Verification items for the finished model (mm, model axes). Face numbers are marked on the shaded views. A direction names the side the tool comes from. Give positions to 0.01 mm unless a question says otherwise; leave off trailing zeros. Loops run counter-clockwise (first coordinate to the right, second up) from the corner with the lowest first, then second, coordinate; pieces in that order, holes last. Notation, with made-up numbers: (16, 37.25) -> (70, 37.25) arc R33 cw to (70, 67.25) -> close; hole circle Ø7 at (44, 56.25). An arc over 180 degrees is marked (long way). Answer in a Markdown table with one row per item. Add a question column.
Q1. Material ranges on probe 1 along X at (y, z) = (38.5, 70.5); probe 2 along Y at (x, z) = (12, 71.6); probe 3 along Z at (x, y) = (-9, 7.5), recorded low to high.
Q2. Section check A-A on y = 8.5. Enter the section's corners in (x, z), and give its area (3 significant figures).
Q3. Section check B-B on x = 12. Enter the section's corners in (y, z), and give its area (3 significant figures).
Q4. Section check C-C on x = 3.5. Enter the section's corners in (y, z).
Q5. Set-up check for the marked faces 5, 6, 7, 8 and 9: record each of +Z, -Z, +X, -X, +Y, -Y from which the full face is reachable in a straight line by a thin tool's end or side.
Q6. Release check for a two-part mould opening along Z. For the marked faces 1, 2, 3 and 4 record: pulls with the +Z half, pulls with the -Z half, needs draft (parallel to the pull), parting line crosses it, or undercut.
Q7. Gauge pin test, flat ends, axial feed: P1, Ø3, axis at x = -13.75, y = 31.4, coming from the -Z side; P2, Ø15, axis at x = -4, y = 12.5, coming from the +Z side; P3, Ø1.5, axis at y = 12.5, z = 67, coming from the +X side; P4, Ø1.4, axis at x = -5.5, z = 71.5, coming from the +Y side. Record the tip position at first contact, or that the pin passes through.
Q8. Section check D-D on z = 61.5. Enter the section's corners in (x, y), and give its area (3 significant figures).
Autodesk Inventor part; units mm, degrees
ref_plane "РабПлоскость2" through (-11.5, 28.8975, 52.6492) normal (0, 0, -1) x (0, 1, 0)
ref_plane "РабПлоскость3" through (-11.5, 28.8975, 52.6492) normal (0, 0, -1) x (0, 1, 0)
ref_plane "РабПлоскость4" through (-15, 28.8975, 52.6492) normal (0, -1, 0) x (1, 0, 0)
ref_plane "РабПлоскость1" through (0, 34.8975, 74.4992) normal (0, 0, -1) x (1, 0, 0)
sketch "Эскиз1" plane through (0, 34.8975, 74.4992) normal (0, 0, -1) x (1, 0, 0)
  line L0 (11.5, 6) -> (11.5, -6)
  line L1 (15, -6) -> (11.5, -6)
  arc A0 (15, -6) -> (16, -5) centre (15, -5) ccw
  line L2 (16, -1.25) -> (16, -5)
  line L3 (14, -1.25) -> (16, -1.25)
  arc A1 (12.8, -0.05) -> (14, -1.25) centre (14, -0.05) ccw
  line L4 (12.8, 0.05) -> (12.8, -0.05)
  arc A2 (14, 1.25) -> (12.8, 0.05) centre (14, 0.05) ccw
  line L5 (16, 1.25) -> (14, 1.25)
  line L6 (16, 5) -> (16, 1.25)
  arc A3 (16, 5) -> (15, 6) centre (15, 5) ccw
  line L7 (11.5, 6) -> (15, 6)
  circle A4 centre (13.75, 3.5) radius 1.25
  circle A5 centre (13.75, -3.5) radius 1.25
  line L8 (-11.5, -6) -> (-11.5, 6)
  line L9 (-15, 6) -> (-11.5, 6)
  arc A6 (-15, 6) -> (-16, 5) centre (-15, 5) ccw
  line L10 (-16, 1.3872) -> (-16, 5)
  line L11 (-14, 1.3872) -> (-16, 1.3872)
  arc A7 (-12.802, 0.1186) -> (-14, 1.3872) centre (-14, 0.1872) ccw
  line L12 (-12.802, 0.0186) -> (-12.802, 0.1186)
  arc A8 (-14, -1.25) -> (-12.802, 0.0186) centre (-14, -0.05) ccw
  line L13 (-16, -1.25) -> (-14, -1.25)
  line L14 (-16, -5) -> (-16, -1.25)
  arc A9 (-16, -5) -> (-15, -6) centre (-15, -5) ccw
  line L15 (-11.5, -6) -> (-15, -6)
  circle A10 centre (-13.75, 3.5) radius 1.25
  circle A11 centre (-13.75, -3.5) radius 1.25
  line L16 (16, 5) -> (16, 6)
  line L17 (16, 6) -> (15, 6)
  line L18 (-16, 5) -> (-16, 6)
  line L19 (-16, 6) -> (-15, 6)
  point P0 (0, 34.8975)
extrude "Выдавливание1" add sketch "Эскиз1" along normal blind 6
sketch "Эскиз2" plane through (0, 34.8975, 68.4992) normal (0, 0, -1) x (-1, 0, 0)
  point P0 (0, -34.8975)
sketch "Эскиз3" plane through (11.5, 28.8975, 74.4992) normal (0, -1, 0) x (1, 0, 0)
  line L0 (4.5, 0) -> (4.5, -6)
  line L1 (4.5, -6) -> (0, -6)
  line L2 (0, -6) -> (0, 0)
  line L3 (0, 0) -> (4.5, 0)
  line L4 (4.5, 0) -> (4.5, -6)
  line L5 (-27.5, 0) -> (-27.5, -6)
  line L6 (-23, 0) -> (-23, -6)
  line L7 (-27.5, -6) -> (-23, -6)
  line L8 (-23, -6) -> (-23, 0)
  line L9 (-23, 0) -> (-27.5, 0)
  line L10 (-27.5, 0) -> (-27.5, -6)
  line L11 (0, -6) -> (-23, -6)
  line L12 (-23, -6) -> (-23, 0)
  line L13 (-23, 0) -> (0, 0)
  line L14 (0, 0) -> (0, -6)
  line L15 (18.5784, -1.45) -> (-41.4216, -1.45)
  point P0 (-11.5, -74.4992)
  point P1 (4.5, -1.45)
  point P2 (-27.5, -1.45)
extrude "Выдавливание2" add sketch "Эскиз3" along normal blind 30 contours L0 L1 L2 L15 | L2 L11 L6 L15 | L6 L7 L5 L15
sketch "Эскиз4" plane through (0, 34.8975, 68.4992) normal (0, 0, -1) x (-1, 0, 0)
  line L0 (-16, -6) -> (-11.5, -6)
  line L1 (16, -6) -> (16, -36)
  line L2 (-16, -6) -> (16, -6)
  line L3 (16, -6) -> (16, -16)
  line L4 (16, -16) -> (-16, -16)
  line L5 (-16, -16) -> (-16, -6)
  point P0 (16, -6)
  point P1 (-11.5, -6)
  dimension "d4" = 10
ref_plane "РабПлоскость2" through (-11.5, 28.8975, 52.6492) normal (0, 0, -1) x (0, 1, 0)
sketch "Эскиз5" plane through (0, 34.8975, 68.4992) normal (0, 0, -1) x (-1, 0, 0)
  line L0 (-16, -36) -> (16, -36)
  line L1 (16, -36) -> (-16, -36)
  line L2 (-16, -36) -> (-16, -32)
  line L3 (-16, -32) -> (16, -32)
  line L4 (16, -32) -> (16, -36)
  point P0 (0, -34.8975)
  point P1 (-16, -36)
  dimension "d7" = 4
ref_plane "РабПлоскость3" through (-11.5, 28.8975, 52.6492) normal (0, 0, -1) x (0, 1, 0)
extrude "Выдавливание4" add sketch "Эскиз5" along normal up to surface (15.85 mm away)
sketch "Эскиз6" plane through (-16, 2.8975, 68.4992) normal (0, 1, 0) x (1, 0, 0)
  line L0 (32, -4.55) -> (32, 15.85)
  line L1 (0, -4.55) -> (0, 15.85)
  line L2 (32, 15.85) -> (0, 15.85)
  line L3 (0, 15.85) -> (0, 11.85)
  line L4 (0, 11.85) -> (32, 11.85)
  line L5 (32, 11.85) -> (32, 15.85)
  point P0 (16, 68.4992)
  point P1 (32, 11.85)
  dimension "d10" = 4
ref_plane "РабПлоскость4" through (-15, 28.8975, 52.6492) normal (0, -1, 0) x (1, 0, 0)
extrude "Выдавливание5" add sketch "Эскиз6" along normal up to surface (26 mm away)
sketch "Эскиз7" plane through (-16, 2.8975, 68.4992) normal (0, 1, 0) x (1, 0, 0)
  line L0 (32, 11.85) -> (0, 11.85)
  line L1 (0, 0) -> (0, 11.85)
  line L2 (32, 0) -> (0, 0)
  line L3 (32, 0) -> (32, 11.85)
  point P0 (16, 68.4992)
sketch "Эскиз8" plane through (-16, 2.8975, 68.4992) normal (0, 1, 0) x (1, 0, 0)
  circle A0 centre (8, 5.925) radius 2
  circle A1 centre (24, 5.925) radius 2
  line L0 (27.5, 0) -> (31, 0)
  line L1 (4.5, 0) -> (27.5, 0)
  line L2 (0, 0) -> (0, 11.85)
  line L3 (32, 0) -> (32, 11.85)
  point P0 (16, 68.4992)
  dimension "d13" = 4
  dimension "d14" = 4
  dimension "d15" = 5.925
  dimension "d16" = 5.925
  dimension "d17" = 8
  dimension "d18" = 8
extrude "Выдавливание6" cut sketch "Эскиз8" against normal blind 10
sketch "Эскиз9" plane through (0, 34.8975, 68.4992) normal (0, 0, -1) x (-1, 0, 0)
  circle A0 centre (-12, -16.8489) radius 2
  circle A1 centre (12, -16.8489) radius 2
  line L0 (-16, -36) -> (-16, -6)
  line L1 (-16, -6) -> (16, -6)
  line L2 (16, -1.3872) -> (16, -32)
  point P0 (0, -34.8975)
  dimension "d21" = 4
  dimension "d22" = 4
  dimension "d24" = 4
  dimension "d25" = 24
extrude "Выдавливание7" cut sketch "Эскиз9" against normal blind 10
properties part number "держатель сервомоторчика"
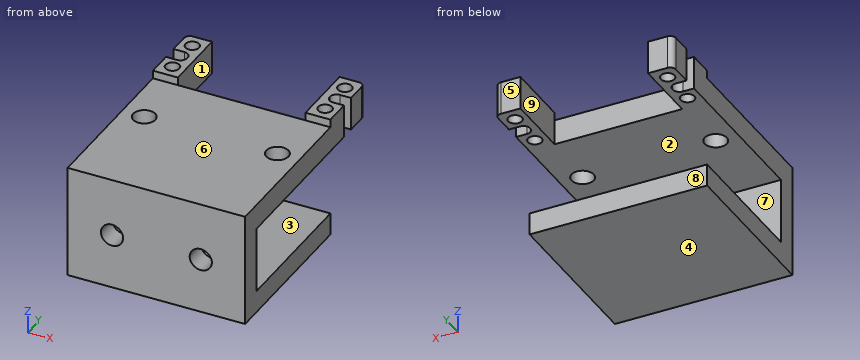
Taken from the geometry:
| question | item | result |
|---|---|---|
| 1 | probe 1 | x = -16 to -15, -12.5 to -11.5, 11.5 to 12.5, 15 to 16 |
| 1 | probe 2 | y = -1.1 to 16.05, 20.05 to 40.9 |
| 1 | probe 3 | z = 52.65 to 56.65, 68.5 to 73.05 |
| 2 | outline | (-16, 52.65) -> (16, 52.65) -> (16, 56.65) -> (-16, 56.65) -> close; (-16, 68.5) -> (16, 68.5) -> (16, 73.05) -> (-16, 73.05) -> close |
| 2 | area | 274 mm² |
| 3 | outline | (-1.1, 52.65) -> (28.9, 52.65) -> (28.9, 56.65) -> (2.9, 56.65) -> (2.9, 68.5) -> (16.05, 68.5) -> (16.05, 73.05) -> (-1.1, 73.05) -> close; (20.05, 68.5) -> (40.9, 68.5) -> (40.9, 74.5) -> (28.9, 74.5) -> (28.9, 73.05) -> (20.05, 73.05) -> close |
| 3 | area | 358 mm² |
| 4 | outline | (-1.1, 52.65) -> (28.9, 52.65) -> (28.9, 56.65) -> (2.9, 56.65) -> (2.9, 68.5) -> (28.9, 68.5) -> (28.9, 73.05) -> (-1.1, 73.05) -> close |
| 5 | face 5 | +Z, -Z, +X, -X, +Y |
| 5 | face 6 | +Z, +X, -X, -Y |
| 5 | face 7 | +X, -X, +Y |
| 5 | face 8 | -Z, +X, -X, +Y |
| 5 | face 9 | +Z, -Z, +Y |
| 6 | face 1 | needs draft |
| 6 | face 2 | undercut |
| 6 | face 3 | undercut |
| 6 | face 4 | pulls with the -Z half |
| 7 | P1 | stops at z = 68.5 |
| 7 | P2 | stops at z = 73.05 |
| 7 | P3 | passes through |
| 7 | P4 | stops at y = 28.9 |
| 8 | outline | (-16, -1.1) -> (-9.69, -1.1) -> (-9.69, 2.9) -> (-16, 2.9) -> close; (-6.31, -1.1) -> (6.31, -1.1) -> (6.31, 2.9) -> (-6.31, 2.9) -> close; (9.69, -1.1) -> (16, -1.1) -> (16, 2.9) -> (9.69, 2.9) -> close |
| 8 | area | 101 mm² |
